Work out the finished part from the listing and answer in its coordinate system (mm). A direction names the side the tool comes from. Round coordinates to 2 decimals unless told otherwise and drop trailing zeros. Write each loop counter-clockwise with the first axis right and the second up, starting at its lowest first coordinate (ties: lowest second). Pieces come first, ordered by that corner, then holes. Notation, with made-up numbers: (47, 58) -> (56, 58) arc R34 ccw to (56, 89) -> close; hole circle Ø9 at (75.25, 88). An arc over 180 degrees is marked (long way). Answer as a JSON object with one key per item and string values. Group by question number.
from build123d import *

# Parameters (mm, degrees)
BOSS_EXTRUDE1_DEPTH       = 4
SKETCH2_R                 = 11.25
CUT_EXTRUDE1_DEPTH        = 9
M4X0_7_TAPPED_HOLE3_D     = 3.3
M4X0_7_TAPPED_HOLE1_D     = 3.3
M4X0_7_TAPPED_HOLE1_DEPTH = 8
M4X0_7_TAPPED_HOLE1_TIP   = 0.991420021
SKETCH6_R                 = 2
CUT_EXTRUDE3_DEPTH        = 8
CHAMFER1_SIZE             = 0.5


with BuildPart() as part:
    # Sketch1 → Boss-Extrude1 (new body, symmetric)
    with BuildSketch(Plane.XY):
        with BuildLine():
            Line((21, 0), (21, 18.4))
            Line((21, 18.4), (-21, 18.4))
            Line((-21, 18.4), (-21, 0))
            ThreePointArc((-21, 0), (-18.076871405, -10.687690125), (-10.121264743, -18.4))
            Line((-10.121264743, -18.4), (10.121264743, -18.4))
            ThreePointArc((10.121264743, -18.4), (18.076871405, -10.687690125), (21, 0))
        make_face()
    extrude(amount=BOSS_EXTRUDE1_DEPTH, both=True)

    # Sketch2 → Cut-Extrude1 (cut, through all)
    with BuildSketch(Plane.XY.offset(4)):
        Circle(SKETCH2_R)
    extrude(amount=-CUT_EXTRUDE1_DEPTH, mode=Mode.SUBTRACT)

    # M4x0.7 Tapped Hole3 (through all)
    with Locations(Plane.XY.offset(4)):
        with Locations((-11.490485194, 11.490485194), (11.490485194, 11.490485194), (11.490485194, -11.490485194), (-11.490485194, -11.490485194)):
            Hole(M4X0_7_TAPPED_HOLE3_D / 2)

    # M4x0.7 Tapped Hole1
    with Locations(Plane(origin=(0, 18.4, 0), x_dir=(1, 0, 0), z_dir=(0, 1, 0))):
        with Locations((-17, 0), (17, 0)):
            Hole(M4X0_7_TAPPED_HOLE1_D / 2, depth=M4X0_7_TAPPED_HOLE1_DEPTH)
            with Locations((0, 0, -(M4X0_7_TAPPED_HOLE1_DEPTH + M4X0_7_TAPPED_HOLE1_TIP / 2))):  # 118° drill point
                Cone(0, M4X0_7_TAPPED_HOLE1_D / 2, M4X0_7_TAPPED_HOLE1_TIP, mode=Mode.SUBTRACT)

    # Sketch6 → Cut-Extrude3 (cut)
    with BuildSketch(Plane(origin=(-3.375, 18.4, 0), x_dir=(0, 0, -1), z_dir=(0, -1, 0))):
        with Locations((0, -13.625)):
            Circle(SKETCH6_R)
        with Locations((0, 20.375)):
            Circle(SKETCH6_R)
    extrude(amount=CUT_EXTRUDE3_DEPTH, mode=Mode.SUBTRACT)

    # Chamfer1
    chamfer1_edges = [part.edges().sort_by_distance(p)[0] for p in [
        (-21, 9.2, 4),
        (-18.076871405, -10.687690125, 4),
        (0, -18.4, 4),
        (-11.25, 0, -4),
        (-11.25, 0, 4),
        (18.076871405, -10.687690125, 4),
        (0, -18.4, -4),
        (-18.076871405, -10.687690125, -4),
        (-21, 9.2, -4),
        (21, 9.2, 4),
        (21, 9.2, -4),
        (18.076871405, -10.687690125, -4),
    ]]
    chamfer(chamfer1_edges, length=CHAMFER1_SIZE)


solid = part.part
1) A cutting plane is placed at A-A on x = 0. Determine the outline of the cut face in (y, z), plus the area to 3 significant figures.
2) Straight lines are drawn through the part: L1, parallel to X at y = 13.25, z = 0; L2, parallel to Y at x = -12, z = -3; L3, parallel to Y at x = 13, z = -0.5. For each, find the intervals that lie inside material, in ascending order.
3) A cutting plane is placed at B-B on z = 1. State how many separate pieces and enclosed holes the cut face has, plus the area to 3 significant figures.
4) Each of these flat-tipped pins is pushed along its axis until it touches: P1, Ø2, axis at x = 17.5, z = -0.5, coming from the +Y side; P2, Ø3, axis at x = 17, z = 0, coming from the -Y side; P3, Ø1.5, axis at y = -8, z = 1.5, coming from the -X side. Where does it stop, or does it pass through?
5) For a pull along Y with two mould halves and no side action, classify faces 3 (the face through (5.19, -9.98, 0.05)), 4 (the face through (17.3, 9.6, 0.1)), 5 (the face through (0, 13, -4)) as released by +Y, released by -Y, zero draft, split by the parting line, or undercut.
6) A tool of negligible diameter and unlimited length cuts with its end or side. For faces 1 (the face through (19, 14, 0)), 2 (the face through (17.684, -10.635, 3.865)), from which of +Z, -Z, +X, -X, +Y, -Y can it reach the whole face along a straight path? Write none if from no direction.
Established:
{
 "1": {"outline": "(-18.4, -3.5) -> (-17.9, -4) -> (-11.75, -4) -> (-11.25, -3.5) -> (-11.25, 3.5) -> (-11.75, 4) -> (-17.9, 4) -> (-18.4, 3.5) -> close; (11.25, -3.5) -> (11.75, -4) -> (18.4, -4) -> (18.4, 4) -> (11.75, 4) -> (11.25, 3.5) -> close", "area": "114 mm²"},
 "2": {"L1": "x = -21 to -19, -15 to 15, 19 to 21", "L2": "y = -17.23 to -13.06, -9.92 to 9.92, 13.06 to 18.4", "L3": "y = -16.49 to -12.16, -10.82 to 10.82, 12.16 to 18.4"},
 "3": {"separate pieces": "1", "enclosed holes": "5", "area": "941 mm²"},
 "4": {"P1": "stops at y = 10.4", "P2": "stops at y = -14.17", "P3": "stops at x = -19.71"},
 "5": {"face 3": "undercut", "face 4": "released by +Y", "face 5": "zero draft"},
 "6": {"face 1": "+Y", "face 2": "+Z, +X, -Y"}
}
